Could you check a few things on this model? Use its own coordinates, in mm. A direction names the side the tool comes from. Give positions to 0.01 mm unless a question says otherwise; leave off trailing zeros. Loops run counter-clockwise (first coordinate to the right, second up) from the corner with the lowest first, then second, coordinate; pieces in that order, holes last.
1. Imagine slicing it at A-A (z = -30.5). List the corners of the cut face in (x, y) for me, plus the area to 3 significant figures.
2. Imagine slicing it at B-B (x = 70). List the corners of the cut face in (y, z) for me, plus the area to 3 significant figures.
3. Imagine slicing it at C-C (y = 3). List the corners of the cut face in (x, z) for me.
4. For P1, Ø9.5, axis at y = 30, z = -41.5, coming from the +X side; P2, Ø21, axis at x = 76, z = -45, coming from the +Y side, each with a flat end and sliding along its axis, tell me the tip position at first contact or that it passes through.
5. I need wall thicknesses on line 1 along X through (y, z) = (9, -30); line 2 along X through (y, z) = (25.5, -33); line 3 along X through (y, z) = (12.5, -36). Which ranges of each line are inside material? Lowest first, please.
6. For faces 1 (the flat face through (91, 7, -30)), 2 (the flat face through (49, 30, -31)), 3 (the flat face through (14, 23, -23)), which set-ups out of +Z, -Z, +X, -X, +Y, -Y let a thin tool reach every point of the face, with its end or its side?
7. Imagine slicing it at D-D (y = 24.5). List the corners of the cut face in (x, z) for me.
8. Thinking about a two-plate mould opening in X: for faces 4 (the flat face through (0, 23, -30)), 5 (the flat face through (25, 23, -46)), 6 (the flat face through (7, 23, 0)), which applies, +X half, -X half, draft (parallel to the pull), parting line (faces both ways), or undercut?
```python
from build123d import *

# Parameters (mm, degrees)
EXTRUDE_1_DEPTH = 46
SKETCH_2_W      = 42
SKETCH_2_H      = 61
SKETCH_2_R      = 10
EXTRUDE_2_DEPTH = 14


with BuildPart() as part:
    # 스케치1 → 보스-돌출1 (new body)
    with BuildSketch(Plane(origin=(0, 0, 0), x_dir=(1, 0, 0), z_dir=(0, 1, 0))):
        Polygon((0, 0), (0, 61), (49, 61), (49, 0), (35, 0), (35, 46), (14, 46), (14, 0), align=None)
    extrude(amount=EXTRUDE_1_DEPTH)

    # 스케치2 → 보스-돌출2 (add)
    with BuildSketch(Plane(origin=(0, 0, 0), x_dir=(1, 0, 0), z_dir=(0, 1, 0))):
        with Locations((70, 30.5)):
            Rectangle(SKETCH_2_W, SKETCH_2_H)
        with Locations(Location((70, 30.5, 0), (0, 0, 270))):
            Circle(SKETCH_2_R, mode=Mode.SUBTRACT)
    extrude(amount=EXTRUDE_2_DEPTH)


solid = part.part
```
Derived:
1. outline: (0, 0) - (14, 0) - (14, 46) - (0, 46) - close; (35, 0) - (60, 0) - (60, 14) - (49, 14) - (49, 46) - (35, 46) - close; (80, 0) - (91, 0) - (91, 14) - (80, 14) - close
1. area: 1,600 mm2
2. outline: (0, -61) - (14, -61) - (14, -40.5) - (0, -40.5) - close; (0, -20.5) - (14, -20.5) - (14, 0) - (0, 0) - close
2. area: 574 mm2
3. outline: (0, -61) - (91, -61) - (91, 0) - (35, 0) - (35, -46) - (14, -46) - (14, 0) - (0, 0) - close; hole circle Ø20 at (70, -30.5)
4. P1: stops at x = 49
4. P2: stops at y = 14
5. line 1: x = 0 to 14, 35 to 60.01, 79.99 to 91
5. line 2: x = 0 to 14, 35 to 49
5. line 3: x = 0 to 14, 35 to 61.65, 78.35 to 91
6. face 1: +Z, -Z, +X, +Y, -Y
6. face 2: +Z, -Z, +X, +Y
6. face 3: +Z, +Y, -Y
7. outline: (0, -61) - (49, -61) - (49, 0) - (35, 0) - (35, -46) - (14, -46) - (14, 0) - (0, 0) - close
8. face 4: -X half
8. face 5: undercut
8. face 6: draft
